Autodesk Inventor part; units mm, degrees
ref_plane "工作平面4" through (-13.0444, 55, -10.5556) normal (-0.9962, 0.0872, 0) x (0, 0, 1)
ref_plane "YZ Plane" through (0, 0, 0) normal (1, 0, 0) x (0, 1, 0)
ref_plane "XZ Plane" through (0, 0, 0) normal (0, 1, 0) x (-1, 0, 0)
sketch "草图1" plane through (0, 0, 0) normal (0, 1, 0) x (-1, 0, 0)
  line L0 (20.0444, 13.4444) -> (-9.9556, 13.4444)
  line L1 (-9.9556, 13.4444) -> (-9.9556, -16.5556)
  line L2 (-9.9556, -16.5556) -> (20.0444, -16.5556)
  line L3 (20.0444, -16.5556) -> (20.0444, 13.4444)
  line L4 (0.0444, 13.4444) -> (-7.4556, 13.4444)
  line L5 (0.0444, 13.4444) -> (7.5444, 13.4444)
  dimension "d0" = 30
  dimension "d1" = 30
extrude "拉伸1" add sketch "草图1" along normal blind 2
sketch "草图2" plane through (0, 2, 0) normal (0, 1, 0) x (1, 0, 0)
  line L0 (9.9556, 16.5556) -> (-20.0444, 16.5556)
  circle A0 centre (4.9556, 12.5556) radius 1.5
  circle A1 centre (-10.0444, 12.5556) radius 1.5
  circle A2 centre (-10.0444, -9.4444) radius 1.5
  circle A3 centre (4.9556, -9.4444) radius 1.5
  line L1 (-10.0444, 12.5556) -> (-10.0444, 16.5556)
  line L2 (4.9556, 12.5556) -> (4.9556, 16.5556)
  line L3 (-10.0444, -9.4444) -> (-10.0444, -13.4444)
  line L4 (-20.0444, -13.4444) -> (9.9556, -13.4444)
  line L5 (4.9556, -9.4444) -> (4.9556, -13.4444)
  line L6 (9.9556, -13.4444) -> (9.9556, 16.5556)
  line L7 (-20.0444, 16.5556) -> (-20.0444, -13.4444)
  point P0 (0, 0)
  dimension "d15" = 3
  dimension "d16" = 3
  dimension "d17" = 3
  dimension "d108" = 4
  dimension "d109" = 4
  dimension "d110" = 4
  dimension "d111" = 4
  dimension "d112" = 5
  dimension "d113" = 10
extrude "拉伸2" cut sketch "草图2" against normal blind 2 contours A0 | A1 | A2 | A3
sketch "草图3" plane through (0, 2, 0) normal (0, 1, 0) x (1, 0, 0)
  circle A0 centre (4.9556, 12.5556) radius 1.5
  circle A1 centre (-10.0444, -9.4444) radius 1.5
  line L0 (2.9556, 10.5556) -> (2.9556, -7.4444)
  line L1 (-13.0444, 10.5556) -> (-13.0444, -7.4444)
  line L2 (-13.0444, -7.4444) -> (2.9556, -7.4444)
  line L3 (-13.0444, 10.5556) -> (2.9556, 10.5556)
  line L4 (-22.598, 1.5556) -> (13.9828, 1.5556)
  point P0 (0, 0)
  dimension "d137" = 11
extrude "拉伸3" add sketch "草图3" along normal blind 53 contours L0 L4 L1 L3 | L0 L2 L1 L4
chamfer "倒角5" distance 16 angle 5 1 edges at (2.9556, 55, -1.5556) measured on face at (-2.3778, 55, 1.4444)
sketch "草图29" plane through (0, 2, 0) normal (0, 1, 0) x (1, 0, 0)
  line L0 (-13.0444, -7.4444) -> (-13.0444, 10.5556)
  line L1 (-13.0444, 10.5556) -> (-20.9964, 10.5556)
  line L2 (-20.9964, 10.5556) -> (-20.9964, -16.1821)
  line L3 (-20.9964, -16.1821) -> (-13.0444, -16.1821)
  line L4 (-13.0444, -16.1821) -> (-13.0444, 10.5556)
  line L5 (-13.0444, 10.5556) -> (-22.8537, 10.5556)
  line L6 (-22.8537, 10.5556) -> (-22.8537, 28.4787)
  line L7 (-22.8537, 28.4787) -> (-13.0444, 28.4787)
  line L8 (-13.0444, 28.4787) -> (-13.0444, 10.5556)
  point P0 (0, 0)
  point P1 (-20.0444, -13.4444)
extrude "拉伸15" cut sketch "草图29" against normal blind 20
sketch "草图31" plane through (-13.0444, 55, 7.4444) normal (0.0872, 0.9962, 0) x (0.9962, -0.0872, 0)
  line L0 (0, 18) -> (0, 0)
  line L1 (0, 9) -> (16.0611, 9)
  line L2 (16.0611, 0) -> (16.0611, 18)
  circle A0 centre (8.0306, 9) radius 1.5
  point P0 (17.7884, 7.4444)
  dimension "d134" = 3
extrude "拉伸16" cut sketch "草图31" against normal blind 20
ref_plane "工作平面4" through (-13.0444, 55, -10.5556) normal (-0.9962, 0.0872, 0) x (0, 0, 1)
ref_plane "工作平面3" through (2.9556, 53.6002, -1.5556) normal (0.0872, 0.9962, 0) x (0.9962, -0.0872, 0)
sketch "草图36" plane through (-13.0444, 55, -10.5556) normal (-0.9962, 0.0872, 0) x (0, 0, 1)
  line L0 (18, 0) -> (0, 0)
  circle A0 centre (9, 0) radius 15
  point P0 (10.5556, -53.6538)
  dimension "d140" = 30
extrude "拉伸17" cut sketch "草图36" against normal blind 200
sketch "草图38" plane through (-13.0444, 55, -10.5556) normal (-0.9962, 0.0872, 0) x (0, 0, 1)
  line L0 (9, -17.5895) -> (9, 63.4105)
  circle A0 centre (9, 22.9105) radius 40.5
  point P0 (10.5556, -53.6538)
  dimension "d143" = 81
extrude "拉伸18" add sketch "草图38" against normal blind 20
sketch "草图39" plane through (-11.0477, 77.8233, -1.5556) normal (-0.9962, 0.0872, 0) x (0, 0, 1)
  line L0 (-48.0605, 0) -> (68.7188, 0)
  line L1 (68.7188, 0) -> (68.7188, 57.1611)
  line L2 (68.7188, 57.1611) -> (-48.0605, 57.1611)
  line L3 (-48.0605, 57.1611) -> (-48.0605, 0)
  point P0 (1.5556, -76.5643)
extrude "拉伸19" cut sketch "草图39" against normal through all
sketch "草图41" plane through (-13.0444, 55, -10.5556) normal (-0.9962, 0.0872, 0) x (0, 0, 1)
  line L0 (49.5, 22.9105) -> (-31.5, 22.9105)
  circle A0 centre (9, 22.9105) radius 40
  point P0 (10.5556, -53.6538)
  dimension "d148" = 80
extrude "拉伸20" cut sketch "草图41" against normal blind 20
equation "\"折弯半径\" = 厚度"
equation "\"折弯释压宽度\" = 厚度"
equation "\"折弯释压深度\" = 0.5 * 厚度"
equation "\"拐角释压尺寸\" = 4 * 厚度"
equation "\"最小余量\" = 2 * 厚度"
equation "\"过渡半径\" = 折弯半径"
equation "\"Jacobi半径尺寸\" = 折弯半径"
equation "\"间隙大小\" = 厚度"
properties part number "_3D 打印"
Could you check a few things on this model? Use its own coordinates, in mm. A direction names the side the tool comes from. Round coordinates to 2 decimals unless told otherwise and drop trailing zeros. Loops run counter-clockwise (first coordinate to the right, second up) from the corner with the lowest first, then second, coordinate; pieces in that order, holes last. Notation, with made-up numbers: (-14, -2) -> (-9, -2) arc R25 ccw to (-9, 14) -> close; hole circle Ø3 at (48.5, 76.25). An arc over 180 degrees is marked (long way). Put each result on its own line as item: value.
Q1. Please list where these lines run through material, in increasing order: line 1 (Z direction, x = 1.5, y = 10); line 2 (Z direction, x = -8.25, y = 63); line 3 (Z direction, x = 3, y = 54.5). Write a range as from..to.
Checks:
line 1: -10.56..7.44
line 2: -39.36..-38.83, 35.71..36.25
line 3: -35.55..-34.96, 31.84..32.44
Q2. For pin 1 Ø9 at (y, z) = (23.5, 2.5) entering from +X; pin 2 Ø0.6 at (x, y) = (3, 1) entering from +Z; pin 3 Ø8 at (x, y) = (0.5, 24.5) entering from +Z, each with a flat end and sliding along its axis, tell me the tip position at first contact or that it passes through.
Checks:
pin 1: x = 2.96
pin 2: z = 13.44
pin 3: z = 7.44
Q3. Thinking about a two-plate mould opening in Z: for faces 5 (the cylindrical face through (-10.24, 1.014, 7.957)), 6 (the flat face through (6.074, 44.047, -25.745)), 7 (the cylindrical face through (-9.24, 1.01, -13.82)), 8 (the flat face through (-5, 20, -10.556)), which applies, pulls with the +Z half, pulls with the -Z half, needs draft (parallel to the pull), parting line crosses it, or undercut?
Checks:
face 5: undercut
face 6: needs draft
face 7: undercut
face 8: pulls with the -Z half
Q4. I want a section at A-A on z = -8. Write out the boundary of the cut face in (x, y), and give its area (3 significant figures).
Checks:
outline: (-14.53, 37.99) -> (-13.04, 37.86) -> (-13.04, 0) -> (9.96, 0) -> (9.96, 2) -> (2.96, 2) -> (2.96, 36.46) -> (5.39, 36.25) -> (5.44, 36.75) -> (-14.49, 38.5) -> close
area: 619 mm2
Q5. I want a section at D-D on z = -17.5. Write out the boundary of the cut face in (x, y), and give its area (3 significant figures).
Checks:
outline: (-14.29, 40.74) -> (5.63, 38.99) -> (5.68, 39.53) -> (-14.24, 41.28) -> close
area: 10.9 mm2
Q6. I want a section at B-B on y = 8.5. Write out the boundary of the cut face in (x, z).
Checks:
outline: (-13.04, -10.56) -> (2.96, -10.56) -> (2.96, 7.44) -> (-13.04, 7.44) -> close
Q7. I want a section at C-C on x = -9.75. Give the number of separate pieces and of enclosed holes in the cut face, and give its area (3 significant figures).
Checks:
separate pieces: 3
enclosed holes: 0
area: 749 mm2
Q8. Which directions (+Z, -Z, +X, -X, +Y, -Y) give clear straight access to the entire face, cutting with the end or side of a thin tool? Please do faces 1 (the flat face through (4, 2, -1)), 2 (the flat face through (-2, 1, 13.444)), 3 (the cylindrical face through (-6.6, 36.78, -1.58)), 4 (the cylindrical face through (4.76, 1.014, 7.957)).
Checks:
face 1: +X
face 2: +Z, +X, -X, -Y
face 3: none
face 4: -Y
